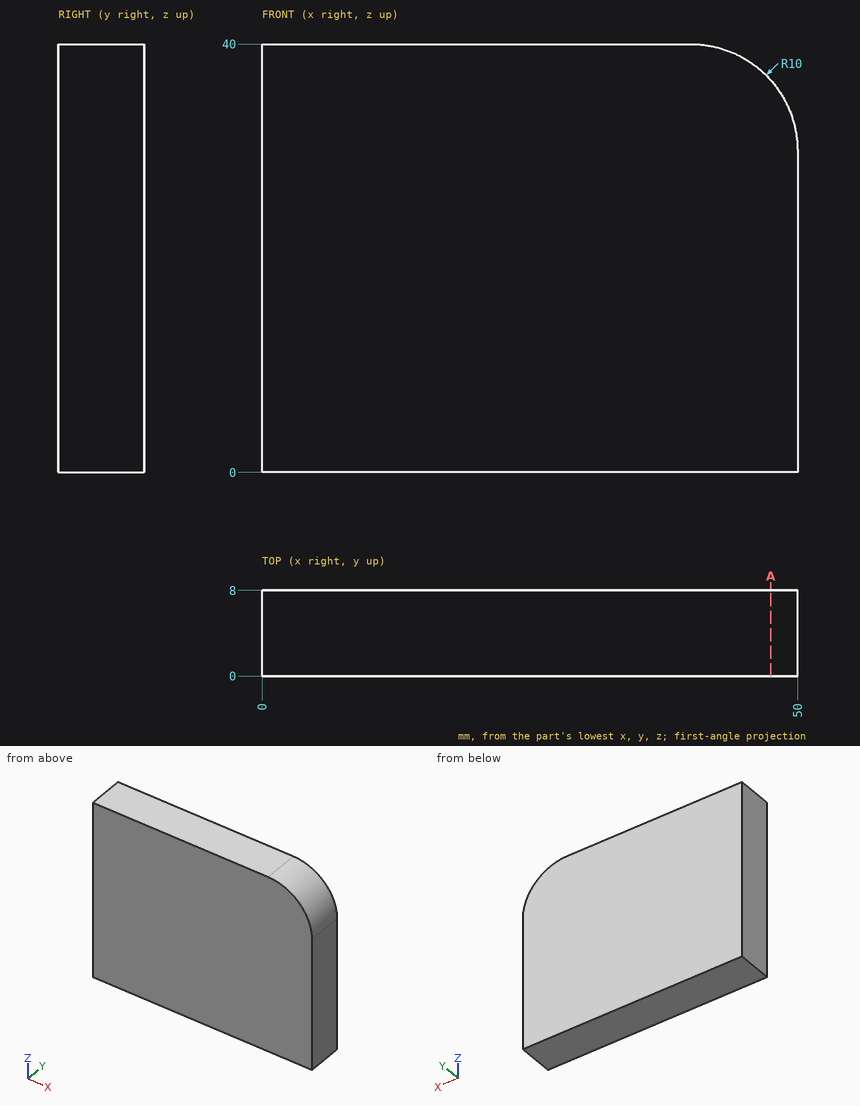
Design review of the part shown in the three views and the two pictorial views. Dimensions are in mm from the part's minimum x, y and z. Round coordinates to 2 decimals unless told otherwise and drop trailing zeros. Loops run counter-clockwise (first coordinate to the right, second up) from the corner with the lowest first, then second, coordinate; pieces in that order, holes last. Notation, with made-up numbers: (-16.75, -11.75) -> (36.25, -11.75) arc R8 cw to (36.25, -0.75) -> close; hole circle Ø10 at (24.25, 41). An arc over 180 degrees is marked (long way). Use one line per item in the form item = value. Start each with the question number.
Q1. Wall thickness on line 1 along Z through (x, y) = (48.5, 2); line 2 along Z through (x, y) = (44.5, 4.5); line 3 along X through (y, z) = (3.5, 30.5): over which ranges is each line inside the solid? List them lowest first. Write a range as [from, to].
Q2. For pin 1 Ø1 at (y, z) = (6, 33.5) entering from +X, flat-tipped, find the tip position at first contact; note if it passes through.
Q3. We need section A-A on x = 47.5. Give the boundary of the cut face in (y, z), then the cut area to 3 significant figures.
Calculated:
q1.line_1 = [0, 35.27]
q1.line_2 = [0, 38.93]
q1.line_3 = [0, 49.99]
q2.pin_1 = 49.54
q3.outline = (0, 0) -> (8, 0) -> (8, 36.61) -> (0, 36.61) -> close
q3.area = 293 mm²
